from build123d import *

# Parameters (mm, degrees)
ESBO_O1_W                = 49
ESBO_O1_H                = 21.976467336
ESBO_O1_R                = 0.750862634
ESBO_O1_W_2              = 11.832091764
ESBO_O1_H_2              = 5.865635034
RESSALTO_EXTRUS_O1_DEPTH = 3
ESBO_O2_W                = 40
ESBO_O2_H                = 21.976467336
ESBO_O2_R                = 5.05
RESSALTO_EXTRUS_O2_DEPTH = 1.8
ESBO_O3_W                = 40
ESBO_O3_H                = 21.97646734
ESBO_O3_R                = 4.05
RESSALTO_EXTRUS_O3_DEPTH = 1.5


with BuildPart() as part:
    # Esboço1 → Ressalto-extrusão1 (new body)
    with BuildSketch(Plane.XY):
        Rectangle(ESBO_O1_W, ESBO_O1_H)
        with Locations((-0.421929048, 4.932817517)):
            Circle(ESBO_O1_R, mode=Mode.SUBTRACT)
        with Locations((7.916045882, 0.729927039)):
            Circle(ESBO_O1_R, mode=Mode.SUBTRACT)
        with Locations(Location((-0.421929048, -4.932817517, 0), (0, 0, 180))):
            Circle(ESBO_O1_R, mode=Mode.SUBTRACT)
        with Locations(Location((-7.916045882, 0.729927039, 0), (0, 0, 180))):
            Circle(ESBO_O1_R, mode=Mode.SUBTRACT)
        Rectangle(ESBO_O1_W_2, ESBO_O1_H_2, mode=Mode.SUBTRACT)
    extrude(amount=RESSALTO_EXTRUS_O1_DEPTH)

    # Esboço2 → Ressalto-extrusão2 (add)
    with BuildSketch(Plane.ZY.offset(24.5)):
        with Locations((20, 0)):
            Rectangle(ESBO_O2_W, ESBO_O2_H)
        with Locations((30, 0)):
            Circle(ESBO_O2_R, mode=Mode.SUBTRACT)
    extrude(amount=RESSALTO_EXTRUS_O2_DEPTH)

    # Esboço3 → Ressalto-extrusão3 (add)
    with BuildSketch(Plane(origin=(24.5, 0, 0), x_dir=(0, 0, -1), z_dir=(1, 0, 0))):
        with Locations((-20, -2e-09)):
            Rectangle(ESBO_O3_W, ESBO_O3_H)
        with Locations((-30, 0)):
            Circle(ESBO_O3_R, mode=Mode.SUBTRACT)
    extrude(amount=RESSALTO_EXTRUS_O3_DEPTH)


solid = part.part
Verification items for the finished model (mm, model axes). A direction names the side the tool comes from. Give positions to 0.01 mm unless a question says otherwise; leave off trailing zeros. Write each loop counter-clockwise with the first axis right and the second up, starting at its lowest first coordinate (ties: lowest second). Pieces come first, ordered by that corner, then holes. Notation, with made-up numbers: (18.5, 39) -> (61.5, 39) arc R18 ccw to (61.5, 74) -> close; hole circle Ø7 at (50.25, -35). An arc over 180 degrees is marked (long way). Use CSV: the item, a comma, the result in double quotes.
(1) Set-up check for faces 1 (the flat face through (5, 5, 3)), 2 (the flat face through (-5.916, 0, 1)), 3 (the flat face through (0, 10.988, 2)): record each of +Z, -Z, +X, -X, +Y, -Y from which the full face is reachable in a straight line by a thin tool's end or side.
Derived:
face 1,"+Z, +Y, -Y"
face 2,"+Z, -Z"
face 3,"+Z, -Z, +X, -X, +Y"
(2) Go/stop test with flat-tipped pins: pin 1 (11 mm diameter, centred on x = -6.5, y = -2.5, fed in from +Z); pin 2 (2 mm diameter, centred on x = 1.5, y = 1.5, fed in from +Z). Record where each tip stops, or that it passes through.
Derived:
pin 1,"stops at z = 3"
pin 2,"passes through"
(3) Sectioned sample at C-C (z = 18.5). Record the cut outline in (x, y).
Derived:
outline,"(-26.3, -10.99) -> (-24.5, -10.99) -> (-24.5, 10.99) -> (-26.3, 10.99) -> close; (24.5, -10.99) -> (26, -10.99) -> (26, 10.99) -> (24.5, 10.99) -> close"
(4) Sectioned sample at B-B (x = 5). Record the cut outline in (y, z), plus the area to 3 significant figures.
Derived:
outline,"(-10.99, 0) -> (-2.93, 0) -> (-2.93, 3) -> (-10.99, 3) -> close; (2.93, 0) -> (10.99, 0) -> (10.99, 3) -> (2.93, 3) -> close"
area,"48.3 mm^2"
(5) Sectioned sample at D-D (x = -12). Record the cut outline in (y, z), plus the area to 3 significant figures.
Derived:
outline,"(-10.99, 0) -> (10.99, 0) -> (10.99, 3) -> (-10.99, 3) -> close"
area,"65.9 mm^2"
(6) Sectioned sample at A-A (z = 30). Record the cut outline in (x, y), plus the area to 3 significant figures.
Derived:
outline,"(-26.3, -10.99) -> (-24.5, -10.99) -> (-24.5, -5.05) -> (-26.3, -5.05) -> close; (-26.3, 5.05) -> (-24.5, 5.05) -> (-24.5, 10.99) -> (-26.3, 10.99) -> close; (24.5, -10.99) -> (26, -10.99) -> (26, -4.05) -> (24.5, -4.05) -> close; (24.5, 4.05) -> (26, 4.05) -> (26, 10.99) -> (24.5, 10.99) -> close"
area,"42.2 mm^2"
(7) Material ranges on L1, parallel to X at y = -7.25, z = 31.5; L2, parallel to Z at x = 10.5, y = 9; L3, parallel to X at y = 2.5, z = 26, recorded low to high.
Derived:
L1,"x = -26.3 to -24.5, 24.5 to 26"
L2,"z = 0 to 3"
L3,"x = 24.5 to 26"
(8) Release check for a two-part mould opening along Z. For faces 4 (the flat face through (25, 0, 40)), 5 (the cylindrical face through (-25.387, 0.222, 24.955)), 6 (the flat face through (5.916, 0, 1)) record: +Z half, -Z half, draft (parallel to the pull), parting line (faces both ways), or undercut.
Derived:
face 4,"+Z half"
face 5,"undercut"
face 6,"draft"
